The model under review builds one solid part; all positions refer to its coordinate system, in mm. A direction names the side the tool comes from. Round coordinates to 2 decimals unless told otherwise and drop trailing zeros. Loops run counter-clockwise (first coordinate to the right, second up) from the corner with the lowest first, then second, coordinate; pieces in that order, holes last. Notation, with made-up numbers: (-1, 12) - (56, 12) arc R5 ccw to (56, 17) - close; hole circle Ø5 at (80, -28.75). An arc over 180 degrees is marked (long way). Answer as CSV lines item,"result".
Autodesk Fusion 360 part; units mm, degrees
sketch "Sketch1" plane through (0, 0, 0) normal (0, 0, 1) x (1, 0, 0)
  line L0 (0, 0) -> (480, 0)
  line L1 (480, 0) -> (480, 100)
  line L2 (480, 100) -> (0, 100)
  line L3 (0, 100) -> (0, 0)
  dimension "d1" = 480
  dimension "d2" = 100
extrude "Extrude1" add sketch "Sketch1" along normal blind 5
sketch "Sketch2" plane through (0, 0, 5) normal (0, 0, 1) x (-1, 0, 0)
  line L0 (0, -100) -> (0, 0)
  line L1 (0, 0) -> (-480, 0)
  line L2 (-480, 0) -> (-480, -100)
  line L3 (-480, -100) -> (0, -100)
  line L4 (0, -100) -> (-5, -100)
  line L5 (-5, -100) -> (-5, 0)
  line L6 (-5, 0) -> (0, 0)
  line L7 (0, 0) -> (0, -100)
  line L8 (-480, -100) -> (-475, -100)
  line L9 (-475, -100) -> (-475, 0)
  line L10 (-475, 0) -> (-480, 0)
  line L11 (-480, 0) -> (-480, -100)
  dimension "d5" = 5
  dimension "d6" = 100
  dimension "d7" = 5
  dimension "d8" = 100
extrude "Extrude2" add sketch "Sketch2" along normal blind 100 contours L0 L1 L3 L4 L5 L6 L7 | L1 L2 L3 L8 L9 L10 L11
sketch "Sketch3" plane through (480, 0, 0) normal (1, 0, 0) x (0, 1, 0)
  line L0 (0, 0) -> (100, 0)
  line L1 (100, 0) -> (100, 105)
  line L2 (100, 105) -> (0, 105)
  line L3 (0, 105) -> (0, 0)
  circle A0 centre (50, 75) radius 15
  dimension "d11" = 30
extrude "Extrude3" cut sketch "Sketch3" against normal blind 500 contours A0
sketch "Sketch4" plane through (0, 0, 5) normal (0, 0, 1) x (-1, 0, 0)
  line L0 (-5, -100) -> (-5, 0)
  line L1 (-5, 0) -> (-475, 0)
  line L2 (-475, 0) -> (-475, -100)
  line L3 (-475, -100) -> (-5, -100)
  circle A0 centre (-50, -50) radius 5
  circle A1 centre (-425, -50) radius 5
  dimension "d14" = 10
  dimension "d15" = 10
extrude "Extrude4" cut sketch "Sketch4" against normal blind 2 contours A0 | A1
sketch "Sketch5" plane through (0, 0, 5) normal (0, 0, 1) x (-1, 0, 0)
  circle A0 centre (-425, -50) radius 5
  circle A1 centre (-50, -50) radius 5
  line L0 (-5, -100) -> (-5, 0)
  line L1 (-5, 0) -> (-475, 0)
  line L2 (-475, 0) -> (-475, -100)
  line L3 (-475, -100) -> (-5, -100)
  circle A2 centre (-50, -50) radius 3
  circle A3 centre (-425, -50) radius 3
  dimension "d18" = 6
  dimension "d19" = 6
extrude "Extrude5" cut sketch "Sketch5" against normal blind 6 contours A2 | A3
fillet "Fillet1" radius 50 4 edges at (477.5, 0, 105) (477.5, 100, 105) (2.5, 100, 105) (2.5, 0, 105)
1. Tool access review of faces 4 (the face through (421.7, 49.9, 3)), 5 (the face through (237, 51, 5)), 6 (the face through (2.54, 15.03, 90.74)): name each direction out of +Z, -Z, +X, -X, +Y, -Y from which nothing blocks a thin tool from reaching the whole face with its end or side.
Numbers:
face 4,"+Z"
face 5,"+Z, +Y, -Y"
face 6,"+Z, +X, -X, -Y"
2. Take a section at D-D (x = 201). State the section outline as (y, z) points.
Numbers:
outline,"(0, 0) - (100, 0) - (100, 5) - (0, 5) - close"
3. Take a section at C-C (y = 92.5). State the section outline as (x, z) points.
Numbers:
outline,"(0, 0) - (480, 0) - (480, 81.35) - (475, 81.35) - (475, 5) - (5, 5) - (5, 81.35) - (0, 81.35) - close"
4. Draft analysis for pull direction Y (two halves, no side actions). For faces 1 (the face through (477.46, 84.97, 90.74)), 2 (the face through (5, 51, 43)), 3 (the face through (54, 47, 4)), state which applies: +Y half, -Y half, draft (parallel to the pull), parting line (faces both ways), or undercut.
Numbers:
face 1,"+Y half"
face 2,"draft"
face 3,"undercut"
5. Take a section at A-A (z = 10). State the section outline as (x, y) points.
Numbers:
outline,"(0, 0) - (5, 0) - (5, 100) - (0, 100) - close; (475, 0) - (480, 0) - (480, 100) - (475, 100) - close"
6. Clearance check with flat-ended pins moving along their axes: pin 1 (3 mm diameter, centred on x = 282, y = 84.5, fed in from +Z); pin 2 (3 mm diameter, centred on x = 51.5, y = 51, fed in from +Z). State where each tip first meets the part, or that it passes through.
Numbers:
pin 1,"stops at z = 5"
pin 2,"stops at z = 3"
7. Wall thickness on probe 1 along X at (y, z) = (50, 1.25); probe 2 along X at (y, z) = (75.5, 43.5); probe 3 along X at (y, z) = (50, 4.6): over which ranges is each line inside the solid? List them lowest first.
Numbers:
probe 1,"x = 0 to 47, 53 to 422, 428 to 480"
probe 2,"x = 0 to 5, 475 to 480"
probe 3,"x = 0 to 45, 55 to 420, 430 to 480"
8. Take a section at B-B (z = 75). State the section outline as (x, y) points, plus the area to 3 significant figures.
Numbers:
outline,"(0, 4.17) - (5, 4.17) - (5, 35) - (0, 35) - close; (0, 65) - (5, 65) - (5, 95.83) - (0, 95.83) - close; (475, 4.17) - (480, 4.17) - (480, 35) - (475, 35) - close; (475, 65) - (480, 65) - (480, 95.83) - (475, 95.83) - close"
area,"617 mm²"
